```python
from build123d import *

# Parameters (mm, degrees)
EXTRUDE009_DEPTH = 4
SKETCH003_R      = 8.31
SKETCH003_R_2    = 6.23
EXTRUDE003_DEPTH = 2


with BuildPart() as obj1:
    # Sketch012 (on Face8 of Extrude002) → Extrude009 (new body)
    with BuildSketch(Plane.XY.offset(2)):
        with BuildLine():
            ThreePointArc((26.8733973411, -32.9252261245), (35.4651440174, -23.4195123738), (40.8333333333, -11.7851130198))
            ThreePointArc((40.8333333333, -11.7851130198), (47.7113101314, -18.8477611751), (56.9484135086, -22.2921021863))
            Line((56.9484135086, -22.2921021863), (26.8733973411, -32.9252261245))
        make_face()
        with BuildLine():
            ThreePointArc((56.9484135086, 22.2921021863), (47.7113101314, 18.8477611751), (40.8333333333, 11.7851130198))
            ThreePointArc((40.8333333333, 11.7851130198), (35.4651440174, 23.4195123738), (26.8733973411, 32.9252261245))
            Line((56.9484135086, 22.2921021863), (26.8733973411, 32.9252261245))
        make_face()
    extrude(amount=EXTRUDE009_DEPTH)


with BuildPart() as tampo:
    # Sketch003 (on Face5 of Cut) → Extrude003 (new body)
    with BuildSketch(Plane.XY.offset(4)):
        with BuildLine():
            ThreePointArc((13.3333333333, 37.7123616633), (-40, 0), (13.3333333333, -37.7123616633))
            Line((66.6666666667, -18.8561808316), (13.3333333333, -37.7123616633))
            ThreePointArc((66.6666666667, -18.8561808316), (80, 0), (66.6666666667, 18.8561808316))
            Line((13.3333333333, 37.7123616633), (66.6666666667, 18.8561808316))
        make_face()
        Circle(SKETCH003_R, mode=Mode.SUBTRACT)
        with Locations((60, 0)):
            Circle(SKETCH003_R_2, mode=Mode.SUBTRACT)
    extrude(amount=EXTRUDE003_DEPTH)

    # Cut003: cut obj1
    add(obj1.part, mode=Mode.SUBTRACT)


solid = tampo.part
```
CAD build for the part. Positions are in the model's coordinates, mm. Round coordinates to 2 decimals unless told otherwise and drop trailing zeros. Order: outer loops, then holes, each group sorted by start corner. A loop starts at its lowest first (then second) coordinate and runs counter-clockwise, first axis right, second up. Notation, with made-up numbers: (21.5, -36) - (58.5, -36) arc R32 ccw to (58.5, 3) - close; hole circle Ø9 at (6.25, -34.75). An arc over 180 degrees is marked (long way). Use CSV: the item, a comma, the result in double quotes. Start each with the question number.
1) Saw through at C-C (x = 0). List the corners of the cut face in (y, z).
2) Saw through at A-A (z = 5). List the corners of the cut face in (x, y).
3) Saw through at D-D (x = 60). List the corners of the cut face in (y, z), and give its area (3 significant figures).
4) Pin check, flat tips, straight feed: pin 1 Ø13.5 at (x, y) = (0, 0) entering from -Z; pin 2 Ø1 at (x, z) = (29.5, 6) entering from +Y. Stop position of each tip, or through.
5) Two-plate mould, pull along Y, no slides. Class faces 1 (the flat face through (61.74, 20.6, 4.99)), 2 (the flat face through (20.198, -35.285, 4.986)), 3 (the cylindrical face through (7.926, 2.496, 4.986)): pulls with the +Y half, pulls with the -Y half, needs draft (parallel to the pull), parting line crosses it, or undercut.
6) Wall check: L1, parallel to X at y = 0.5, z = 4.95; L2, parallel to Y at x = 0, z = 5.45; L3, parallel to X at y = 7.5, z = 5.15. Give the ranges that are in metal, low to high. Write a range as [from, to].
7) Saw through at B-B (y = 0). List the corners of the cut face in (x, z).
Values follow:
1,outline,"(-40, 4) - (-8.31, 4) - (-8.31, 6) - (-40, 6) - close; (8.31, 4) - (40, 4) - (40, 6) - (8.31, 6) - close"
2,outline,"(13.33, -37.71) - (26.87, -32.93) arc R42.5 ccw to (40.83, -11.79) arc R22.5 ccw to (56.95, -22.29) - (66.67, -18.86) arc R20 ccw to (66.67, 18.86) - (56.95, 22.29) arc R22.5 ccw to (40.83, 11.79) arc R42.5 ccw to (26.87, 32.93) - (13.33, 37.71) arc R40 ccw (long way) to start; hole circle Ø16.62 at (0, 0); hole circle Ø12.46 at (60, 0)"
3,outline,"(-21.21, 4) - (-6.23, 4) - (-6.23, 6) - (-21.21, 6) - close; (6.23, 4) - (21.21, 4) - (21.21, 6) - (6.23, 6) - close"
3,area,"59.9 mm2"
4,pin 1,"passes through"
4,pin 2,"stops at y = 31.07"
5,face 1,"pulls with the +Y half"
5,face 2,"pulls with the -Y half"
5,face 3,"undercut"
6,L1,"x = [-40, -8.29], [8.29, 53.79], [66.21, 79.99]"
6,L2,"y = [-40, -8.31], [8.31, 40]"
6,L3,"x = [-39.29, -3.58], [3.58, 78.54]"
7,outline,"(-40, 4) - (-8.31, 4) - (-8.31, 6) - (-40, 6) - close; (8.31, 4) - (53.77, 4) - (53.77, 6) - (8.31, 6) - close; (66.23, 4) - (80, 4) - (80, 6) - (66.23, 6) - close"
